The model under review builds one solid part; all positions refer to its coordinate system, in mm. A direction names the side the tool comes from. Round coordinates to 2 decimals unless told otherwise and drop trailing zeros. Write each loop counter-clockwise with the first axis right and the second up, starting at its lowest first coordinate (ties: lowest second). Pieces come first, ordered by that corner, then holes. Notation, with made-up numbers: M 6,86.5 L 41,86.5 A15 cw 41,91.5 Z; hole C 76,73 d7. An arc over 180 degrees is marked long. One line per item, written item: value. Start each with the question number.
1) Take a section at D-D, the plane z = 2.5. Write out the cut boundary in (x, y).
2) Wall thickness on probe 1 along Z at (x, y) = (-20.6, 22.6) (3 decimals); probe 2 along Z at (x, y) = (7, 0.5); probe 3 along X at (y, z) = (14, -8): over which ranges is each line inside the solid? List them lowest first.
3) Take a section at B-B, the plane x = 7. Write out the cut boundary in (y, z).
4) For P1, Ø10, axis at x = -1.5, z = -0.5, coming from the +Y side, flat-tipped, find the tip position at first contact; note if it passes through.
5) Tool access review of faces 4 (the face through (20.99, 16.005, 7.228)), 5 (the face through (0, 0, 0)), 6 (the face through (-20.99, 21.56, -7.66)), 7 (the face through (0, 1.5, 0)): name each direction out of +Z, -Z, +X, -X, +Y, -Y from which nothing blocks a thin tool from reaching the whole face with its end or side.
6) Mouldability with a two-part tool opening along Y and no side actions: class faces 1 (the face through (0, 1, 10)), 2 (the face through (-20.99, 6.615, 8.089)), 3 (the face through (20.99, 34.815, -9.699)) as +Y half, -Y half, draft (parallel to the pull), parting line (faces both ways), or undercut.
7) Take a section at C-C, the plane y = 24.5. Write out the cut boundary in (x, z), and give its area (3 significant figures).
8) Take a section at A-A, the plane y = 28.2. Write out the cut boundary in (x, z).
Autodesk Inventor part; units mm, degrees
ref_plane "YZ Plane" through (0, 0, 0) normal (1, 0, 0) x (0, 1, 0)
ref_plane "XZ Plane" through (0, 0, 0) normal (0, 1, 0) x (-1, 0, 0)
ref_plane "XY Plane" through (0, 0, 0) normal (0, 0, 1) x (1, 0, 0)
sketch "Sketch1" plane through (0, 0, 0) normal (0, 1, 0) x (-1, 0, 0)
  line L0 (20.25, -10) -> (-20.25, -10)
  line L1 (-20.25, -10) -> (-20.25, 10)
  line L2 (-20.25, 10) -> (20.25, 10)
  line L3 (20.25, 10) -> (20.25, -10)
  point P0 (0, 0)
  dimension "d0" = 40.5
  dimension "d1" = 20
  dimension "d2" = 10
  dimension "d3" = 20.25
extrude "Plate1" add sketch "Sketch1" along normal blind 1.5
sketch "Sketch2" plane through (21.75, 0, -10) normal (-1, 0, 0) x (0, -1, 0)
  line L0 (0, 20) -> (0, 0)
  line L1 (0, 0) -> (-45, 0)
  line L2 (-45, 0) -> (-45, 20)
  line L3 (-45, 20) -> (0, 20)
edge flange "Flange1" height 45 angle 90 thickness 1.5 bend radius 0.31 thickness toward (-1, 0, 0) relief tear relief width 1.5 relief depth 0.75 edges at (20.25, 1.5, 0) wall of the first edge with corners at (21.75, 0, 10) (21.75, 0, -10) (21.75, 45, -10) (21.75, 45, 10)
bend "Bend1"
corner "Corner1"
sketch "Sketch3" plane through (-21.75, 0, 10) normal (1, 0, 0) x (0, 1, 0)
  line L0 (0, -20) -> (0, 0)
  line L1 (0, 0) -> (45, 0)
  line L2 (45, 0) -> (45, -20)
  line L3 (45, -20) -> (0, -20)
edge flange "Flange2" height 45 angle 90 thickness 1.5 bend radius 0.31 thickness toward (1, 0, 0) relief tear relief width 1.5 relief depth 0.75 edges at (-20.25, 1.5, 0) wall of the first edge with corners at (-21.75, 0, -10) (-21.75, 0, 10) (-21.75, 45, 10) (-21.75, 45, -10)
bend "Bend2"
corner "Corner2"
sketch "Sketch4" plane through (21.75, 45, 10) normal (1, 0, 0) x (0, 0, -1)
  circle A0 centre (10, -9.9) radius 6.4
  line L0 (0, 0) -> (20, 0)
  line L1 (20, 0) -> (20, -43.19)
  point P0 (10, -45)
  dimension "d25" = 9.9
  dimension "d26" = 12.8
  dimension "d27" = 10
extrude "Extrusion1" cut sketch "Sketch4" against normal blind 50
sketch "Sketch5" plane through (21.75, 45, 10) normal (1, 0, 0) x (0, 0, -1)
  circle A0 centre (10, -9.9) radius 6.4
  line L0 (0, 0) -> (20, 0)
  line L1 (-4, 0) -> (24, 0)
  line L2 (24, 0) -> (24, -9.9)
  line L3 (24, -9.9) -> (-4, -9.9)
  line L4 (-4, -9.9) -> (-4, 0)
  line L5 (0, -43.19) -> (0, 0)
  point P0 (10, -45)
  dimension "d30" = 9.9
  dimension "d31" = 28
  dimension "d32" = 4
extrude "Extrusion2" cut sketch "Sketch5" against normal blind 50 contours L3 A0 | A0 L3 L5 L0 L1 L2 | L3 L4 L1 L5 picked at (9.2435, -7.9053)
fillet "Fillet1" radius 1 4 edges at (-21, 35.1, 10) (-21, 35.1, -10) (21, 35.1, -10) (21, 35.1, 10)
sketch "Sketch8" plane through (0, 0, 0) normal (0, -1, 0) x (1, 0, 0)
  circle A0 centre (8, -8) radius 1.05
  circle A1 centre (-8, -8) radius 1.05
  circle A2 centre (8, 8) radius 1.05
  circle A3 centre (-8, 8) radius 1.05
  circle A4 centre (-7, -7) radius 1.5
  line L0 (-9.33, -10.07) -> (7.53, -10.07)
  line L1 (10.07, -8.5) -> (10.07, 29.6)
  circle A5 centre (7, -7) radius 1.5
  circle A6 centre (-7, 7) radius 1.5
  circle A7 centre (7, 7) radius 1.5
  point P0 (0, 0)
  dimension "d71" = 7
  dimension "d72" = 7
  dimension "d73" = 3
  dimension "d76" = 14
  dimension "d79" = 14
hole "Hole3" at (-7, 0, -7) at (-7, 0, 7) at (7, 0, 7) at (7, 0, -7) direction (0, 1, 0) diameter 3 depth 1.5
sketch "Sketch9" plane through (-21.75, 1.81, -10) normal (-1, 0, 0) x (0, 0, 1)
  circle A0 centre (17.525, 20.79) radius 0.7835
  circle A1 centre (17.525, 5.69) radius 0.7835
  circle A2 centre (2.475, 20.79) radius 0.7835
  circle A3 centre (2.475, 5.69) radius 0.7835
  point P0 (10, -1.81)
hole "Hole4" at (-21.75, 7.5, 7.525) at (-21.75, 7.5, -7.525) at (-21.75, 22.6, -7.525) at (-21.75, 22.6, 7.525) direction (1, 0, 0) diameter 2.1 depth 1.5
sketch "Sketch10" plane through (21.75, 1.81, 10) normal (1, 0, 0) x (0, 0, -1)
  circle A0 centre (3, 13.17) radius 0.7835
  circle A1 centre (10, 5.87) radius 0.7835
  circle A2 centre (17, 13.17) radius 0.7835
  circle A3 centre (2, 26.39) radius 0.7835
  circle A4 centre (18, 26.39) radius 0.7835
  point P0 (10, -1.81)
hole "Hole5" at (21.75, 28.2, 8) at (21.75, 28.2, -8) at (21.75, 14.98, -7) at (21.75, 7.68, 0) at (21.75, 14.98, 7) direction (-1, 0, 0) diameter 2.1 depth 1.5
equation "\"d55\" = Thickness"
equation "\"d62\" = Thickness"
equation "\"d69\" = Thickness"
equation "\"d4\" = Thickness"
equation "\"d5\" = BendReliefWidth"
equation "\"d6\" = BendReliefDepth"
equation "\"d7\" = MinimumRemnant"
equation "\"d8\" = TransitionRadius"
equation "\"d11\" = BendRadius"
equation "\"d12\" = CornerReliefSize"
equation "\"d13\" = GapSize"
equation "\"d14\" = JacobiRadiusSize"
equation "\"d15\" = BendReliefWidth"
equation "\"d16\" = BendReliefDepth"
equation "\"d17\" = MinimumRemnant"
equation "\"d18\" = TransitionRadius"
equation "\"d21\" = BendRadius"
equation "\"d22\" = CornerReliefSize"
equation "\"d23\" = GapSize"
equation "\"d24\" = JacobiRadiusSize"
equation "\"BendReliefWidth\" = Thickness"
equation "\"BendReliefDepth\" = 0.5 * Thickness"
equation "\"CornerReliefSize\" = 4 * Thickness"
equation "\"MinimumRemnant\" = 2 * Thickness"
equation "\"TransitionRadius\" = BendRadius"
equation "\"JacobiRadiusSize\" = BendRadius"
equation "\"GapSize\" = Thickness"
properties part number "axis_10_top_frame" material "Aluminum 6061-AHC"
Checked values:
1. outline: M -21.75,1.81 A1.81 ccw -19.94,0 L 19.94,0 A1.81 ccw 21.75,1.81 L 21.75,29.21 L 20.25,29.21 L 20.25,1.81 A0.31 cw 19.94,1.5 L -19.94,1.5 A0.31 cw -20.25,1.81 L -20.25,29.21 L -21.75,29.21 Z
2. probe 1: z = -10 to -8.575, -6.475 to 6.475, 8.575 to 10
2. probe 2: z = -10 to -8.5, -5.5 to 5.5, 8.5 to 10
2. probe 3: x = -21.75 to -20.25, 20.25 to 21.75
3. outline: M 0,-10 L 1.5,-10 L 1.5,-8.5 L 0,-8.5 Z; M 0,-5.5 L 1.5,-5.5 L 1.5,5.5 L 0,5.5 Z; M 0,8.5 L 1.5,8.5 L 1.5,10 L 0,10 Z
4. P1: stops at y = 1.5
5. face 4: +X
5. face 5: +Z, -Z, +X, -X, -Y
5. face 6: -X
5. face 7: +Z, -Z, +Y
6. face 1: draft
6. face 2: undercut
6. face 3: +Y half
7. outline: M -21.75,-10 L -20.25,-10 L -20.25,10 L -21.75,10 Z; M 20.25,-10 L 21.75,-10 L 21.75,10 L 20.25,10 Z
7. area: 60.0 mm2
8. outline: M -21.75,-10 L -20.25,-10 L -20.25,10 L -21.75,10 Z; M 20.25,-10 L 21.75,-10 L 21.75,-9.05 L 20.25,-9.05 Z; M 20.25,-6.95 L 21.75,-6.95 L 21.75,6.95 L 20.25,6.95 Z; M 20.25,9.05 L 21.75,9.05 L 21.75,10 L 20.25,10 Z
